Could you check a few things on this drawing? It's one solid part, dimensions in mm from its lowest x, y, z. A direction names the side the tool comes from. Coordinates: 2 decimals unless noted, no trailing zeros. Loops run counter-clockwise (first coordinate to the right, second up) from the corner with the lowest first, then second, coordinate; pieces in that order, holes last. Notation, with made-up numbers: (73, 13) -> (125, 13) arc R11 cw to (125, 28) -> close; hole circle Ø4 at (-9, 42.25). An arc over 180 degrees is marked (long way). One line per question, with ' | ' between items.
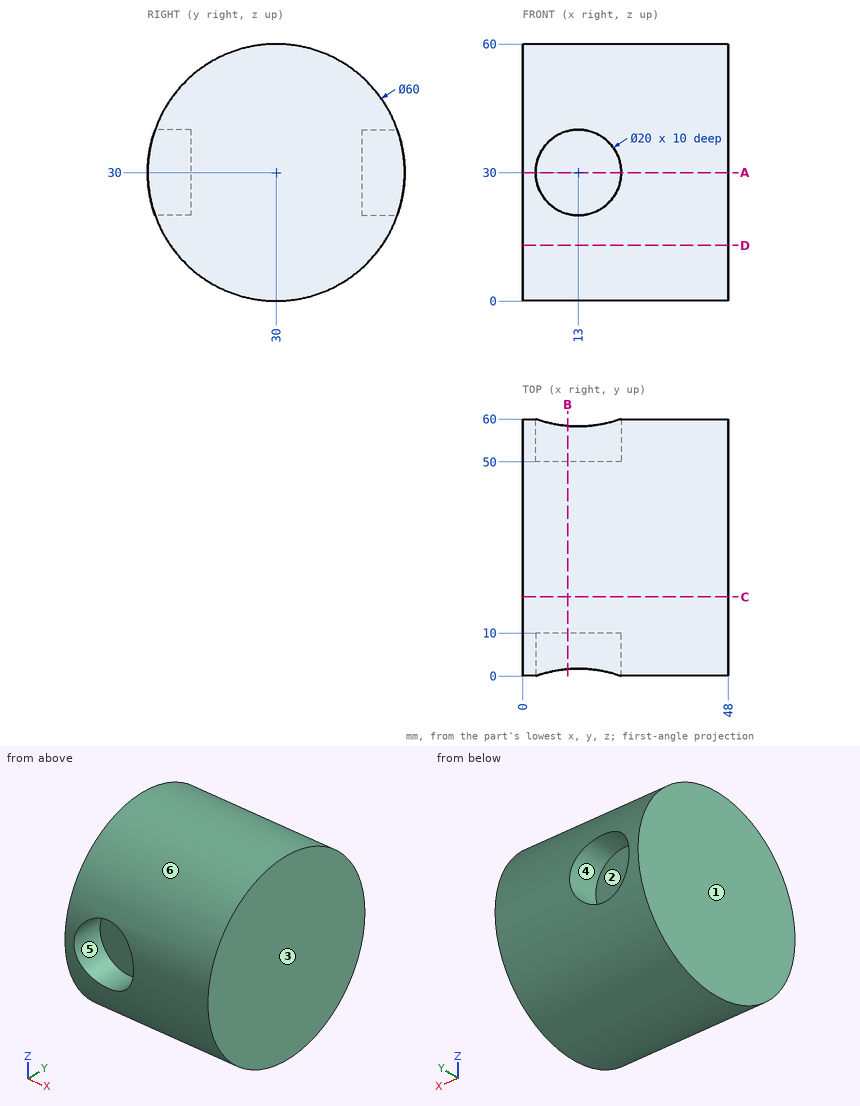
1) On a 3-axis mill with a long thin cutter (end or side, diameter ignored), from which of +Z, -Z, +X, -X, +Y, -Y can I reach the whole of each face in a straight line? I mean the marked faces 4, 5 and 6. Say none if no direction works.
Data:
face 4: +Y | face 5: -Y | face 6: +X, -X
2) If we section it at A-A on z = 30: Please give me the cut outline in (x, y).
Data:
outline: (0, 0) -> (3, 0) -> (3, 10) -> (23, 10) -> (23, 0) -> (48, 0) -> (48, 60) -> (23, 60) -> (23, 50) -> (3, 50) -> (3, 60) -> (0, 60) -> close
3) We'd pull the mould along X, two halves only. Please class the marked faces 1, 2 and 3: pulls with the +X half, pulls with the -X half, needs draft (parallel to the pull), parting line crosses it, or undercut.
Data:
face 1: pulls with the -X half | face 2: undercut | face 3: pulls with the +X half
4) I need wall thicknesses on line 1 along Z through (x, y) = (13, 55.5); line 2 along Z through (x, y) = (13, 6.25); line 3 along Y through (x, z) = (6, 28.5). Which ranges of each line are inside material? Lowest first, please. Write a range as from..to.
Data:
line 1: 14.2..20, 40..45.8 | line 2: 11.67..20, 40..48.33 | line 3: 10..50
5) If we section it at B-B on x = 10.5: Please give me the cut outline in (y, z), and give its area (3 significant figures).
Data:
outline: (1.61, 20.32) arc R30 ccw to (58.39, 20.32) -> (50, 20.32) -> (50, 39.68) -> (58.39, 39.68) arc R30 ccw to (1.61, 39.68) -> (10, 39.68) -> (10, 20.32) -> close | area: 2,460 mm²
6) I'm going to push flat-ended pins straight in: pin 1 Ø4 at (x, z) = (37.5, 36) entering from +Y; pin 2 Ø16 at (x, z) = (12, 30.5) entering from +Y; pin 3 Ø4 at (x, z) = (26, 33) entering from +Y. Where does each tip first touch, or does it pass through?
Data:
pin 1: y = 59.73 | pin 2: y = 50 | pin 3: y = 59.98
7) If we section it at D-D on z = 13: Please give me the cut outline in (x, y), and give its area (3 significant figures).
Data:
outline: (0, 5.28) -> (48, 5.28) -> (48, 54.72) -> (0, 54.72) -> close | area: 2,370 mm²
8) If we section it at C-C on y = 18.5: Please give me the cut outline in (x, z).
Data:
outline: (0, 2.29) -> (48, 2.29) -> (48, 57.71) -> (0, 57.71) -> close
